```python
from build123d import *

# Parameters (mm, degrees)
F0_W     = 40
F0_H     = 40
F1_DEPTH = 3
F2_W     = 40
F2_H     = 5
F3_DEPTH = 7
F4_R     = 19.99999
F5_SIZE  = 2


# Not quite as in the source:
# - a fillet or chamfer is up to 0.001 mm smaller than in the source, because OpenCascade refuses the exact size


with BuildPart() as f1:
    # F0 (on Top) → F1 (new body)
    with BuildSketch(Plane.XY):
        Rectangle(F0_W, F0_H)
    extrude(amount=F1_DEPTH)

    # F2 (on face) → F3 (join)
    with BuildSketch(Plane(origin=(0, 0, 0), x_dir=(1, 0, 0), z_dir=(0, 0, -1))):
        with Locations((0, 17.5)):
            Rectangle(F2_W, F2_H)
        with Locations((0, -17.5)):
            Rectangle(F2_W, F2_H)
    extrude(amount=F3_DEPTH)

    # F4 (radius 20 in the source; OpenCascade refuses exactly that, so slightly less here)
    f4_edges = [f1.edges().sort_by_distance(p)[0] for p in [
        (-20, 20, -2),
        (-20, -20, -2),
    ]]
    fillet(f4_edges, radius=F4_R)

    # F5
    f5_edges = [f1.edges().sort_by_distance(p)[0] for p in [
        (-14.142139, -14.142139, 3),
        (20, -20, -2),
        (20, 0, 3),
        (20, 20, -2),
        (20, 15, -3.5),
        (20, -15, -3.5),
    ]]
    chamfer(f5_edges, length=F5_SIZE)


solid = f1.part
```
CAD build for the part. Positions are in the model's coordinates, mm. A direction names the side the tool comes from. Coordinates: 2 decimals unless noted, no trailing zeros. Order: outer loops, then holes, each group sorted by start corner. A loop starts at its lowest first (then second) coordinate and runs counter-clockwise, first axis right, second up. Notation, with made-up numbers: M 53,30 L 77,30 A13 ccw 77,46 Z; hole C 89,-16.75 d9. An arc over 180 degrees is marked long. Write each question's results on one line, items separated by ' | '. Start each with the question number.
Q1. Pull direction Y, two halves, no side cores. Call faces 4 (the flat face through (0, 0, 0)), 5 (the flat face through (19, 0, 2)), 6 (the conical face through (-12.957, -12.675, 2.875)), 7 (the flat face through (18.8, 18.6, 1.6)): +Y half, -Y half, draft (parallel to the pull), parting line (faces both ways), or undercut.
Q2. Cut at A-A (z = -4.5). List the corners of the cut face in (x, y).
Q3. Flat gauge pins, fed straight in: P1, Ø1.5, axis at y = 14.5, z = 2, coming from the -X side; P2, Ø6, axis at x = -10.5, z = -3, coming from the +Y side; P3, Ø1.5, axis at x = 3.5, y = 9, coming from the -Z side. Where does each tip first touch, or does it go through?
Q4. Which spindle directions (+Z, -Z, +X, -X, +Y, -Y) get a long thin tool onto all of the face, cutting with end or side? Do faces 1 (the flat face through (19, -16, -3)), 2 (the cylindrical face through (-8.651, 18.032, -3.056)), 3 (the flat face through (2, -15, -3)). Say none if no direction does.
Q5. Drill centre lines: probe 1 along Y at (x, z) = (5.5, -2.5); probe 2 along Z at (x, y) = (-5, -14.5); probe 3 along Y at (x, z) = (-12, -3.5). Where is each one in solid material? Low to high. Write a range as from..to.
Q6. Cut at B-B (x = 5). List the corners of the cut face in (y, z).
Found:
1) face 4: undercut | face 5: draft | face 6: -Y half | face 7: +Y half
2) outline: M -13.23,-15 A20 ccw 0,-20 L 18,-20 L 20,-18 L 20,-17 L 18,-15 Z; M -13.23,15 L 18,15 L 20,17 L 20,18 L 18,20 L 0,20 A20 ccw Z
3) P1: x = -13.67 | P2: y = 18.54 | P3: z = 0
4) face 1: -Z, +X | face 2: +Z, -Z, -X, +Y | face 3: -Z, +X, -X
5) probe 1: -20..-15, 15..20 | probe 2: 0..3 | probe 3: -16..-15, 15..16
6) outline: M -20,-7 L -15,-7 L -15,0 L 15,0 L 15,-7 L 20,-7 L 20,1 L 18,3 L -18,3 L -20,1 Z
